from build123d import *

# Parameters (mm, degrees)
F0_W     = 20
F0_H     = 3
F1_DEPTH = 250
F3_DEPTH = 10
F2_R     = 5
F4_DEPTH = 3
F5_R     = 0.5
F7_DEPTH = 25
F8_R     = 0.5


with BuildPart() as f1:
    # F0 (on Front) → F1 (new body, symmetric)
    with BuildSketch(Plane.XZ):
        Rectangle(F0_W, F0_H)
    extrude(amount=F1_DEPTH, both=True)

    # F3 (add): a face of the model
    f3_faces = [f1.faces().sort_by_distance(p)[0] for p in [
        (0, 250, 0),
    ]]
    extrude(f3_faces, amount=F3_DEPTH)

    # F2 (on face) → F4 (cut)
    with BuildSketch(Plane.XY.offset(1.5)):
        with BuildLine():
            ThreePointArc((5, -215), (-3.5355339059, -211.4644660941), (0, -220))
            ThreePointArc((0, -220), (3.5355339059, -218.5355339059), (5, -215))
        make_face()
        with BuildLine():
            ThreePointArc((0, -230), (-5, -235), (0, -240))
            ThreePointArc((0, -240), (3.5355339059, -238.5355339059), (5, -235))
            ThreePointArc((5, -235), (3.5355339059, -231.4644660941), (0, -230))
        make_face()
        with BuildLine():
            ThreePointArc((5, 245), (3.5355339059, 248.5355339059), (0, 250))
            ThreePointArc((0, 250), (-3.5355339059, 241.4644660941), (5, 245))
        make_face()
        with Locations((0, -195)):
            Circle(F2_R)
        with Locations((0, -175)):
            Circle(F2_R)
        with Locations((0, -155)):
            Circle(F2_R)
        with Locations((0, -135)):
            Circle(F2_R)
        with Locations((0, -115)):
            Circle(F2_R)
        with Locations((0, -95)):
            Circle(F2_R)
        with Locations((0, -75)):
            Circle(F2_R)
        with Locations((0, -55)):
            Circle(F2_R)
        with Locations((0, -35)):
            Circle(F2_R)
        with Locations((0, -15)):
            Circle(F2_R)
        with Locations((0, 5)):
            Circle(F2_R)
        with Locations((0, 25)):
            Circle(F2_R)
        with Locations((0, 45)):
            Circle(F2_R)
        with Locations((0, 65)):
            Circle(F2_R)
        with Locations((0, 85)):
            Circle(F2_R)
        with Locations((0, 105)):
            Circle(F2_R)
        with Locations((0, 125)):
            Circle(F2_R)
        with Locations((0, 145)):
            Circle(F2_R)
        with Locations((0, 165)):
            Circle(F2_R)
        with Locations((0, 185)):
            Circle(F2_R)
        with Locations((0, 205)):
            Circle(F2_R)
        with Locations((0, 225)):
            Circle(F2_R)
    extrude(amount=-F4_DEPTH, mode=Mode.SUBTRACT)

    # F5
    f5_edges = [f1.edges().sort_by_distance(p)[0] for p in [
        (10, -250, 0),
        (10, 5, -1.5),
        (10, 260, 0),
        (10, 5, 1.5),
        (0, -250, 1.5),
        (-10, -250, 0),
        (0, -250, -1.5),
        (-10, 5, 1.5),
        (0, 260, 1.5),
        (-10, 260, 0),
        (0, 260, -1.5),
    ]]
    fillet(f5_edges, radius=F5_R)

    # F6 (on face) → F7 (cut)
    with BuildSketch(Plane(origin=(0, 0, -1.5), x_dir=(1, 0, 0), z_dir=(0, 0, -1))):
        Polygon((0, 185), (16.080936417, 185), (32.4585177004, 259.3803107738), (-14.6508449689, 254.37900424), (-14.6508449689, 185), align=None)
    extrude(amount=-F7_DEPTH, mode=Mode.SUBTRACT)

    # F8
    f8_edges = [f1.edges().sort_by_distance(p)[0] for p in [
        (9.853553, -185, -1.353553),
        (10, -185, 0),
        (9.853553, -185, 1.353553),
        (0, -185, 1.5),
        (-9.853553, -185, 1.353553),
        (-10, -185, -0.25),
        (-0.25, -185, -1.5),
    ]]
    fillet(f8_edges, radius=F8_R)


solid = f1.part
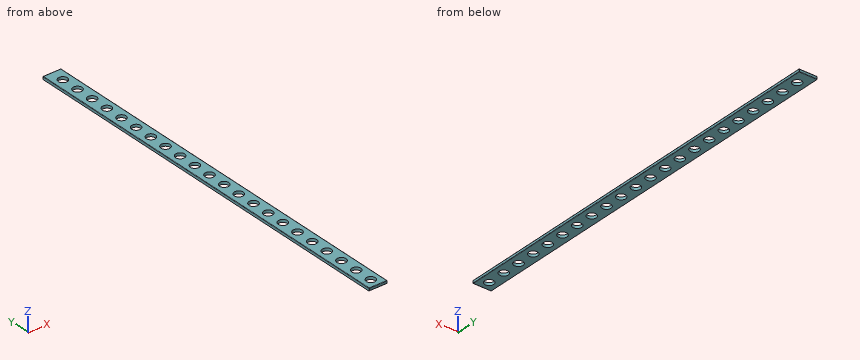
The listing builds one solid part. Answer for the finished solid, in the listing's coordinates (mm). Give positions to 0.01 mm unless a question says otherwise; leave off trailing zeros. Loops run counter-clockwise (first coordinate to the right, second up) from the corner with the lowest first, then second, coordinate; pieces in that order, holes last.
Item 1: Find the intervals of material crossed by line 1 along X through (y, z) = (245, -0.3); line 2 along X through (y, z) = (83.5, 1.1), in increasing order.
Derived:
line 1: x = -10 to -5, 5 to 10
line 2: x = -9.99 to -4.77, 4.77 to 9.99
Item 2: A cutting plane is placed at B-B (z = 0.5). Give the number of separate pieces and of enclosed holes in the cut face, then the cut area to 3 significant figures.
Derived:
separate pieces: 1
enclosed holes: 22
area: 7,170 mm2
Item 3: This flat-tipped pin is pushed along its axis until it touches: pin 1 Ø8 at (x, y) = (0, -175) entering from -Z. Where does it stop, or does it pass through?
Derived:
pin 1: passes through
Item 4: A cutting plane is placed at A-A (y = -95). Give the vertices of the cut face in (x, z).
Derived:
outline: (-10, -1.5) - (-5, -1.5) - (-5, 1.5) - (-9.5, 1.5) arc R0.5 ccw to (-10, 1) - close; (5, -1.5) - (9.5, -1.5) arc R0.5 ccw to (10, -1) - (10, 1) arc R0.5 ccw to (9.5, 1.5) - (5, 1.5) - close
